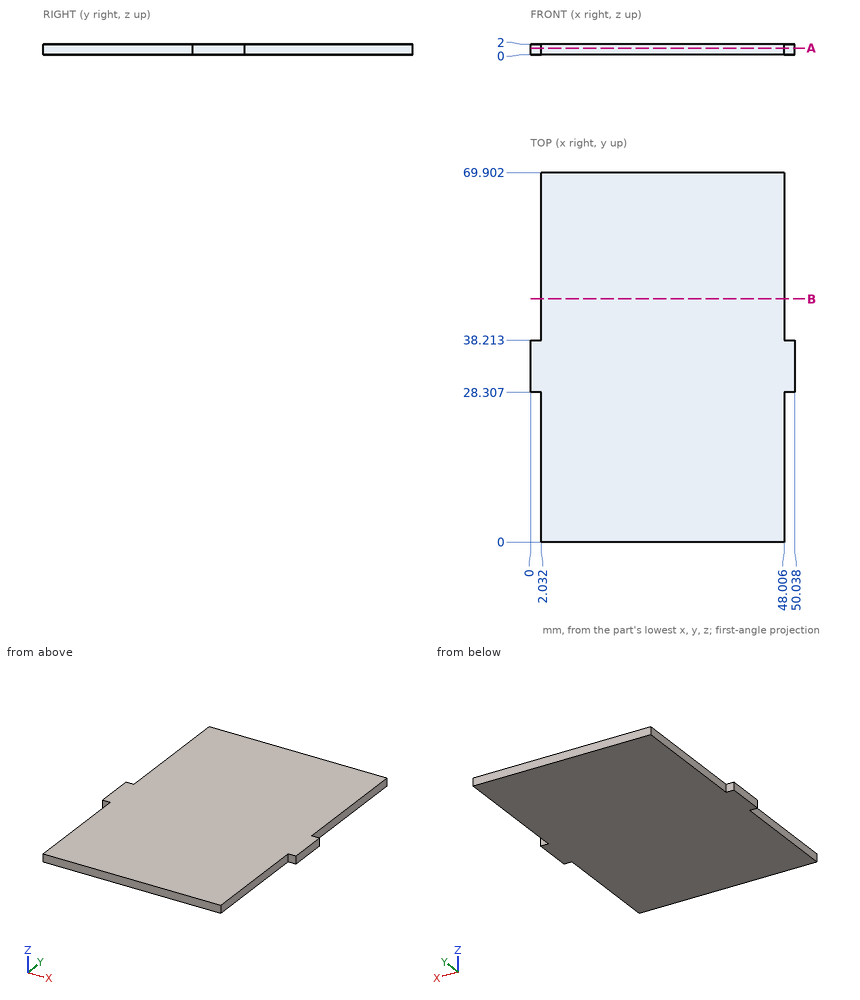
Study the drawing (mm; zero at the part's minimum x, y, z) and answer. Round coordinates to 2 decimals unless told otherwise and drop trailing zeros. Write each loop counter-clockwise with the first axis right and the second up, starting at its lowest first coordinate (ties: lowest second). Pieces come first, ordered by that corner, then holes. Notation, with made-up numbers: (18, -25.5) - (23, -25.5) arc R36 cw to (23, 8.5) - close; hole circle Ø4 at (81.5, -31). An arc over 180 degrees is marked (long way). Use a Markdown table: item, result. Add a question column.
1. Consider line 1 (X direction, y = 62, z = 1.5); line 2 (Y direction, x = 48.5, z = 0.2). Determine where each line is inside the solid, lowest interval first.
2. The part is cut by section B-B (y = 46). Write down the section's boundary in (x, z).
3. The part is cut by section A-A (z = 1.2). Write down the section's boundary in (x, y), and give its area (3 significant figures).
4. Flat-ended cylindrical pins translate along their axes: P1, Ø1, axis at y = 56, z = 0.5, coming from the -X side; P2, Ø1, axis at x = 49, z = 1, coming from the -Y side; P3, Ø1, axis at y = 9.5, z = 0.5, coming from the +X side. Find the tip coordinate at first contact, or state that the pin passes through.
Reported:
| question | item | result |
|---|---|---|
| 1 | line 1 | 2.03 to 48.01 |
| 1 | line 2 | 28.31 to 38.21 |
| 2 | outline | (2.03, 0) - (48.01, 0) - (48.01, 2) - (2.03, 2) - close |
| 3 | outline | (0, 28.31) - (2.03, 28.31) - (2.03, 0) - (48.01, 0) - (48.01, 28.31) - (50.04, 28.31) - (50.04, 38.21) - (48.01, 38.21) - (48.01, 69.9) - (2.03, 69.9) - (2.03, 38.21) - (0, 38.21) - close |
| 3 | area | 3,250 mm^2 |
| 4 | P1 | x = 2.03 |
| 4 | P2 | y = 28.31 |
| 4 | P3 | x = 48.01 |
